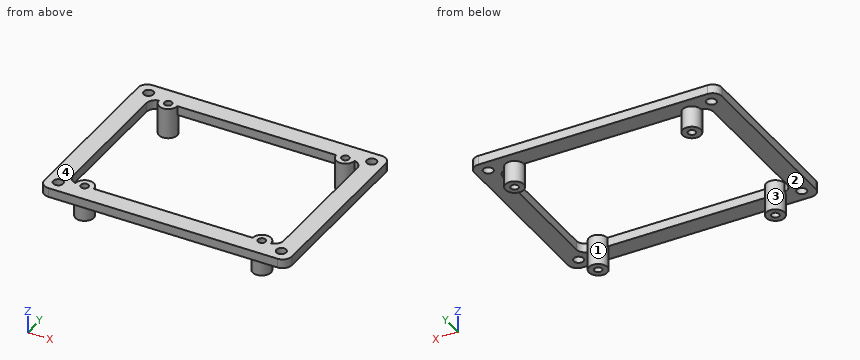
```python
from build123d import *

# Parameters (mm, degrees)
SKETCH1_W           = 81
SKETCH1_H           = 61
SKETCH1_W_2         = 69
SKETCH1_H_2         = 49
EXTRUDE_THIN1_DEPTH = 3
SKETCH2_R           = 1.6
CUT_EXTRUDE1_DEPTH  = 3
FILLET1_R           = 3
SKETCH4_R           = 3
BOSS_EXTRUDE1_DEPTH = 10
CUT_EXTRUDE2_REACH  = 12
SKETCH5_R           = 1.25


with BuildPart() as part:
    # Sketch1 → Extrude-Thin1 (new body)
    with BuildSketch(Plane.XY):
        Rectangle(SKETCH1_W, SKETCH1_H)
        Rectangle(SKETCH1_W_2, SKETCH1_H_2, mode=Mode.SUBTRACT)
    extrude(amount=EXTRUDE_THIN1_DEPTH)

    # Sketch2 → Cut-Extrude1 (cut)
    with BuildSketch(Plane.XY.offset(3)):
        with Locations((-36.5, 26.5)):
            Circle(SKETCH2_R)
        with Locations((36.5, 26.5)):
            Circle(SKETCH2_R)
        with Locations((36.5, -26.5)):
            Circle(SKETCH2_R)
        with Locations((-36.5, -26.5)):
            Circle(SKETCH2_R)
    extrude(amount=-CUT_EXTRUDE1_DEPTH, mode=Mode.SUBTRACT)

    # Fillet1
    fillet1_edges = [part.edges().sort_by_distance(p)[0] for p in [
        (-34.5, 24.5, 1.5),
        (-34.5, -24.5, 1.5),
        (34.5, -24.5, 1.5),
        (34.5, 24.5, 1.5),
        (-40.5, 30.5, 1.5),
        (40.5, 30.5, 1.5),
        (40.5, -30.5, 1.5),
        (-40.5, -30.5, 1.5),
    ]]
    fillet(fillet1_edges, radius=FILLET1_R)

    # Sketch4 → Boss-Extrude1 (add)
    with BuildSketch(Plane.XY.offset(3)):
        with Locations((-29, 24.5)):
            Circle(SKETCH4_R)
        with Locations((29, 24.5)):
            Circle(SKETCH4_R)
        with Locations((29, -24.5)):
            Circle(SKETCH4_R)
        with Locations((-29, -24.5)):
            Circle(SKETCH4_R)
    extrude(amount=-BOSS_EXTRUDE1_DEPTH)

    # Sketch5 → Cut-Extrude2 (cut, up to next)
    with BuildSketch(Plane(origin=(0, 0, -7), x_dir=(-1, 0, 0), z_dir=(0, 0, -1)), mode=Mode.PRIVATE) as cut_extrude2_sk1:
        with Locations((-29, 24.5)):
            Circle(SKETCH5_R)
    cut_extrude2_tool1 = extrude(cut_extrude2_sk1.sketch, amount=-CUT_EXTRUDE2_REACH, mode=Mode.PRIVATE) & part.part
    add(cut_extrude2_tool1.solids().sort_by_distance((29, 24.5, -7))[0], mode=Mode.SUBTRACT)
    # Sketch5 → Cut-Extrude2 (cut, up to next)
    with BuildSketch(Plane(origin=(0, 0, -7), x_dir=(-1, 0, 0), z_dir=(0, 0, -1)), mode=Mode.PRIVATE) as cut_extrude2_sk2:
        with Locations((29, 24.5)):
            Circle(SKETCH5_R)
    cut_extrude2_tool2 = extrude(cut_extrude2_sk2.sketch, amount=-CUT_EXTRUDE2_REACH, mode=Mode.PRIVATE) & part.part
    add(cut_extrude2_tool2.solids().sort_by_distance((-29, 24.5, -7))[0], mode=Mode.SUBTRACT)
    # Sketch5 → Cut-Extrude2 (cut, up to next)
    with BuildSketch(Plane(origin=(0, 0, -7), x_dir=(-1, 0, 0), z_dir=(0, 0, -1)), mode=Mode.PRIVATE) as cut_extrude2_sk3:
        with Locations((-29, -24.5)):
            Circle(SKETCH5_R)
    cut_extrude2_tool3 = extrude(cut_extrude2_sk3.sketch, amount=-CUT_EXTRUDE2_REACH, mode=Mode.PRIVATE) & part.part
    add(cut_extrude2_tool3.solids().sort_by_distance((29, -24.5, -7))[0], mode=Mode.SUBTRACT)
    # Sketch5 → Cut-Extrude2 (cut, up to next)
    with BuildSketch(Plane(origin=(0, 0, -7), x_dir=(-1, 0, 0), z_dir=(0, 0, -1)), mode=Mode.PRIVATE) as cut_extrude2_sk4:
        with Locations((29, -24.5)):
            Circle(SKETCH5_R)
    cut_extrude2_tool4 = extrude(cut_extrude2_sk4.sketch, amount=-CUT_EXTRUDE2_REACH, mode=Mode.PRIVATE) & part.part
    add(cut_extrude2_tool4.solids().sort_by_distance((-29, -24.5, -7))[0], mode=Mode.SUBTRACT)


solid = part.part
```
Verification items for the finished model (mm, model axes). Face numbers are marked on the shaded views. A direction names the side the tool comes from. Round coordinates to 2 decimals unless told otherwise and drop trailing zeros. Loops run counter-clockwise (first coordinate to the right, second up) from the corner with the lowest first, then second, coordinate; pieces in that order, holes last. Notation, with made-up numbers: (-17, 23) -> (14, 23) arc R29 ccw to (14, 44) -> close; hole circle Ø5 at (15, -11.5). An arc over 180 degrees is marked (long way). Answer as a JSON object with one key per item and string values.
Q1. Go/stop test with a flat-tipped pin: P1, Ø4, axis at x = -36.5, y = 26.5, coming from the -Z side. Record where the tip stops, or that it passes through.
Data:
{"P1": "stops at z = 0"}
Q2. Section check D-D (x = 29). Record the boundary of the cut face in (y, z), then the cut area to 3 significant figures.
Data:
{"outline": "(-30.5, 0) -> (-27.5, 0) -> (-27.5, -7) -> (-25.75, -7) -> (-25.75, 3) -> (-30.5, 3) -> close; (-23.25, -7) -> (-21.5, -7) -> (-21.5, 3) -> (-23.25, 3) -> close; (21.5, -7) -> (23.25, -7) -> (23.25, 3) -> (21.5, 3) -> close; (25.75, -7) -> (27.5, -7) -> (27.5, 0) -> (30.5, 0) -> (30.5, 3) -> (25.75, 3) -> close", "area": "88.0 mm2"}
Q3. Section check B-B (x = -17). Record the boundary of the cut face in (y, z).
Data:
{"outline": "(-30.5, 0) -> (-24.5, 0) -> (-24.5, 3) -> (-30.5, 3) -> close; (24.5, 0) -> (30.5, 0) -> (30.5, 3) -> (24.5, 3) -> close"}
Q4. Scan lines: line 1 (Y direction, x = 36.5, z = 0.85); line 2 (Y direction, x = 29, z = -2); line 3 (X direction, y = 5, z = 1.75). Record each from-to range of solid material in increasing order. Write a range as from..to.
Data:
{"line 1": "y = -30.5..-28.1, -24.9..24.9, 28.1..30.5", "line 2": "y = -27.5..-25.75, -23.25..-21.5, 21.5..23.25, 25.75..27.5", "line 3": "x = -40.5..-34.5, 34.5..40.5"}
Q5. Access from +Z, -Z, +X, -X, +Y, -Y to the whole of each face (thin tool, end or side, straight path). Record for the marked faces 3 and 4.
Data:
{"face 3": "-Z", "face 4": "+Z, +X, -X, +Y, -Y"}
Q6. Section check A-A (z = -1.75). Record the boundary of the cut face in (x, y), then the cut area to 3 significant figures.
Data:
{"outline": "circle Ø6 at (-29, -24.5); circle Ø6 at (-29, 24.5); circle Ø6 at (29, -24.5); circle Ø6 at (29, 24.5); hole circle Ø2.5 at (-29, -24.5); hole circle Ø2.5 at (-29, 24.5); hole circle Ø2.5 at (29, -24.5); hole circle Ø2.5 at (29, 24.5)", "area": "93.5 mm2"}
Q7. Section check C-C (y = -20.5). Record the boundary of the cut face in (x, z), then the cut area to 3 significant figures.
Data:
{"outline": "(-40.5, 0) -> (-34.5, 0) -> (-34.5, 3) -> (-40.5, 3) -> close; (34.5, 0) -> (40.5, 0) -> (40.5, 3) -> (34.5, 3) -> close", "area": "36.0 mm2"}
Q8. Draft check along Y on the marked faces 1 and 2. Enter one of: pulls with the +Y half, pulls with the -Y half, needs draft (parallel to the pull), parting line crosses it, or undercut.
Data:
{"face 1": "undercut", "face 2": "needs draft"}
